Source: CAD feature listing. Evaluate the final solid. Frame: model axes, mm. A direction names the side the tool comes from. Give positions to 0.01 mm unless a question says otherwise; leave off trailing zeros. Loops run counter-clockwise (first coordinate to the right, second up) from the corner with the lowest first, then second, coordinate; pieces in that order, holes last. Notation, with made-up numbers: (25.5, 34.5) -> (33.5, 34.5) arc R27 cw to (33.5, 51.5) -> close; hole circle Ø4 at (-29, 43.5). An arc over 180 degrees is marked (long way). Answer as a JSON object with one key per item and string values. Group by question number.
from build123d import *

# Parameters (mm, degrees)
BOSS_EXTRUDE1_DEPTH = 10
SKETCH5_R           = 1.75
CUT_EXTRUDE2_DEPTH  = 38.286056375


with BuildPart() as part:
    # Sketch3 → Boss-Extrude1 (new, symmetric)
    with BuildSketch(Plane(origin=(0, 0, 0), x_dir=(0, 0, -1), z_dir=(1, 0, 0))):
        Polygon((0, -14), (0, -22.5), (-30, -22.5), (-30, 22.5), (0, 22.5), (0, 14), (-2, 14), (-2, 20.5), (-28, 20.5), (-28, -20.5), (-2, -20.5), (-2, -14), align=None)
    extrude(amount=BOSS_EXTRUDE1_DEPTH, both=True)

    # Sketch5 → Cut-Extrude2 (cut, through all)
    with BuildSketch(Plane.XY.offset(2)):
        with Locations((0, -17)):
            Circle(SKETCH5_R)
        with Locations(Location((0, 17, 0), (0, 0, 180))):
            Circle(SKETCH5_R)
    extrude(amount=-CUT_EXTRUDE2_DEPTH, mode=Mode.SUBTRACT)


solid = part.part
(1) Section query D-D on y = -14.5. Return the cut outline in (x, z).
(2) Access query for faces 1 (the face through (0, -22.5, 15)), 2 (the face through (0.228, 15.265, 1.014)), 3 (the face through (0, -14, 1)), 4 (the face through (-10, -3.2, 28.3)), 5 (the face through (0, 0, 28)). Directions: +Z, -Z, +X, -X, +Y, -Y. A direction counts if a zero-diameter tool reaches every point of the face in a straight line with its end or side. Return the directions, or none.
(3) Section query C-C on y = 17. Return the cut outline in (x, z), plus the area to 3 significant figures.
(4) Material intervals for line 1 (Y direction, x = 0, z = 1.5); line 2 (Y direction, x = -8, z = 12.25); line 3 (X direction, y = 17, z = 1.4), sorted ascending. Write a range as from..to.
(5) Section query B-B on z = 24. Return the cut outline in (x, y).
(6) Mould query, pull axis Z, two halves, no side actions, for faces 6 (the face through (0, 19, 2)), 7 (the face through (0, -19, 0)), 8 (the face through (10, -3.2, 28.3)). Classes: pulls with the +Z half, pulls with the -Z half, needs draft (parallel to the pull), parting line crosses it, or undercut.
(7) Section query A-A on x = 0. Return the cut outline in (y, z), plus the area to 3 significant figures.
(8) First-contact query: pin 1 (10 mm diameter, centred on x = 4.5, y = 0.5, fed in from -Z). Flat tip, straight axial feed; report the tip coordinate or a pass-through.
Result:
{
 "1": {"outline": "(-10, 0) -> (10, 0) -> (10, 2) -> (-10, 2) -> close; (-10, 28) -> (10, 28) -> (10, 30) -> (-10, 30) -> close"},
 "2": {"face 1": "+Z, -Z, +X, -X, -Y", "face 2": "-Z", "face 3": "-Z, +X, -X", "face 4": "+Z, -Z, -X, +Y, -Y", "face 5": "+X, -X"},
 "3": {"outline": "(-10, 0) -> (-1.75, 0) -> (-1.75, 2) -> (-10, 2) -> close; (-10, 28) -> (10, 28) -> (10, 30) -> (-10, 30) -> close; (1.75, 0) -> (10, 0) -> (10, 2) -> (1.75, 2) -> close", "area": "73.0 mm²"},
 "4": {"line 1": "-22.5..-18.75, -15.25..-14, 14..15.25, 18.75..22.5", "line 2": "-22.5..-20.5, 20.5..22.5", "line 3": "-10..-1.75, 1.75..10"},
 "5": {"outline": "(-10, -22.5) -> (10, -22.5) -> (10, -20.5) -> (-10, -20.5) -> close; (-10, 20.5) -> (10, 20.5) -> (10, 22.5) -> (-10, 22.5) -> close"},
 "6": {"face 6": "undercut", "face 7": "pulls with the -Z half", "face 8": "needs draft"},
 "7": {"outline": "(-22.5, 0) -> (-18.75, 0) -> (-18.75, 2) -> (-20.5, 2) -> (-20.5, 28) -> (20.5, 28) -> (20.5, 2) -> (18.75, 2) -> (18.75, 0) -> (22.5, 0) -> (22.5, 30) -> (-22.5, 30) -> close; (-15.25, 0) -> (-14, 0) -> (-14, 2) -> (-15.25, 2) -> close; (14, 0) -> (15.25, 0) -> (15.25, 2) -> (14, 2) -> close", "area": "214 mm²"},
 "8": {"pin 1": "z = 28"}
}
